```python
from build123d import *

# Parameters (mm, degrees)
EXTRUDE_1_DEPTH     = 153
EXTRUDE_2_DEPTH     = 1.5
SKETCH_3_W          = 140
SKETCH_3_H          = 3
EXTRUDE_3_DEPTH     = 1.5
EXTRUDE_4_DEPTH     = 8
SKETCH_5_R          = 2.1
CUT_EXTRUDE_1_DEPTH = 4.2


with BuildPart() as part:
    # Эскиз1 → Бобышка-Вытянуть1 (new body)
    with BuildSketch(Plane.XY):
        Polygon((-70, 1), (-70, 95), (70, 95), (70, 1), (68.5, 1), (68.5, 0), (67, 0), (67, 92), (-67, 92), (-67, 0), (-68.5, 0), (-68.5, 1), align=None)
    extrude(amount=EXTRUDE_1_DEPTH)

    # Эскиз2 → Бобышка-Вытянуть2 (add)
    with BuildSketch(Plane(origin=(0, 0, 0), x_dir=(-1, 0, 0), z_dir=(0, 0, -1))):
        Polygon((-70, 92), (-70, 95), (70, 95), (70, 93), (70, 92), (67, 92), (67, 93), (-67, 93), (-67, 92), align=None)
    extrude(amount=EXTRUDE_2_DEPTH)

    # Эскиз3 → Бобышка-Вытянуть3 (add)
    with BuildSketch(Plane(origin=(0, 0, -1.5), x_dir=(-1, 0, 0), z_dir=(0, 0, -1))):
        with Locations((0, 93.5)):
            Rectangle(SKETCH_3_W, SKETCH_3_H)
    extrude(amount=EXTRUDE_3_DEPTH)

    # Эскиз4 → Бобышка-Вытянуть4 (add)
    with BuildSketch(Plane.XY.offset(153)):
        with BuildLine():
            Line((-67, 92), (-60, 92))
            Line((-60, 92), (-60, 89.2))
            ThreePointArc((-60, 89.2), (-61.230151519, 86.230151519), (-64.2, 85))
            Line((-64.2, 85), (-67, 85))
            Line((-67, 85), (-67, 92))
        make_face()
        with BuildLine():
            Line((60, 92), (60, 89.2))
            ThreePointArc((60, 89.2), (61.230151519, 86.230151519), (64.2, 85))
            Line((64.2, 85), (67, 85))
            Line((67, 85), (67, 92))
            Line((67, 92), (60, 92))
        make_face()
    extrude(amount=-EXTRUDE_4_DEPTH)

    # Эскиз5 → Вырез-Вытянуть1 (cut)
    with BuildSketch(Plane.XY.offset(153)):
        with Locations((-65, 90)):
            Circle(SKETCH_5_R)
        with Locations(Location((65, 90, 0), (0, 0, 180))):
            Circle(SKETCH_5_R)
    extrude(amount=-CUT_EXTRUDE_1_DEPTH, mode=Mode.SUBTRACT)


solid = part.part
```
Input: part model. Units: mm. Frame: model coordinates. A direction names the side the tool comes from. Round coordinates to 2 decimals unless told otherwise and drop trailing zeros. Order: outer loops, then holes, each group sorted by start corner. A loop starts at its lowest first (then second) coordinate and runs counter-clockwise, first axis right, second up. Notation, with made-up numbers: (9.25, 80.25) - (24.25, 80.25) arc R19 ccw to (24.25, 94.25) - close; hole circle Ø10 at (30.5, -0.5). An arc over 180 degrees is marked (long way). Answer in a Markdown table with one row per item.
Item 1: Pin query (flat end, axial travel): pin 1 (1.4 mm diameter, centred on x = -65, z = 148.5, fed in from -Y); pin 2 (5.5 mm diameter, centred on x = -65, y = 87.5, fed in from -Z); pin 3 (0.8 mm diameter, centred on x = -4.5, z = -1, fed in from -Y); pin 4 (6.5 mm diameter, centred on x = -65, y = 90, fed in from -Z). Return the tip coordinate at first contact, or that it passes through.
Model answer:
| item | result |
|---|---|
| pin 1 | stops at y = 85 |
| pin 2 | stops at z = 0 |
| pin 3 | stops at y = 93 |
| pin 4 | stops at z = -3 |
Item 2: Line query: line 1 (X direction, y = 46.5, z = 64); line 2 (Y direction, x = -65, z = 151.7); line 3 (Y direction, x = -51, z = 102). Output: solid intervals per line, ascending.
Model answer:
| item | result |
|---|---|
| line 1 | x = -70 to -67, 67 to 70 |
| line 2 | y = 85 to 87.9, 92.1 to 95 |
| line 3 | y = 92 to 95 |
Item 3: Section query B-B (z = 43). Return the cut outline in (x, y), then the cut area to 3 significant figures.
Model answer:
| item | result |
|---|---|
| outline | (-70, 1) - (-68.5, 1) - (-68.5, 0) - (-67, 0) - (-67, 92) - (67, 92) - (67, 0) - (68.5, 0) - (68.5, 1) - (70, 1) - (70, 95) - (-70, 95) - close |
| area | 969 mm² |
Item 4: Section query A-A (y = 16). Return the cut outline in (x, z).
Model answer:
| item | result |
|---|---|
| outline | (-70, 0) - (-67, 0) - (-67, 153) - (-70, 153) - close; (67, 0) - (70, 0) - (70, 153) - (67, 153) - close |
Item 5: Mould query, pull axis X, two halves, no side actions, for faces 5 (the flat face through (1, 95, 76)), 6 (the flat face through (63, 89, 145)), 7 (the cylindrical face through (-61.2, 86.26, 149.06)), 8 (the flat face through (-70, 47, 76)). Classes: released by +X, released by -X, zero draft, split by the parting line, or undercut.
Model answer:
| item | result |
|---|---|
| face 5 | zero draft |
| face 6 | undercut |
| face 7 | undercut |
| face 8 | released by -X |
Item 6: Reachability of faces 1 (the flat face through (0, 93, 153)), 2 (the flat face through (-63, 89, 145)), 3 (the flat face through (-65, 90, 148.8)), 4 (the cylindrical face through (61.2, 86.26, 149.06)) from +Z, -Z, +X, -X, +Y, -Y: full face, straight path, thin tool, end or side. Return the list, or none.
Model answer:
| item | result |
|---|---|
| face 1 | +Z, +X, -X, +Y, -Y |
| face 2 | -Z, -Y |
| face 3 | +Z |
| face 4 | +Z, -Z, -Y |
Item 7: Section query C-C (x = 21.5). Return the cut outline in (y, z).
Model answer:
| item | result |
|---|---|
| outline | (92, -3) - (95, -3) - (95, 153) - (92, 153) - (92, 0) - (93, 0) - (93, -1.5) - (92, -1.5) - close |
